Autodesk Inventor part; units mm, degrees
ref_plane "YZ Plane" through (0, 0, 0) normal (1, 0, 0) x (0, 1, 0)
ref_plane "XZ Plane" through (0, 0, 0) normal (0, 1, 0) x (-1, 0, 0)
ref_plane "XY Plane" through (0, 0, 0) normal (0, 0, 1) x (1, 0, 0)
sketch "Sketch1" plane through (0, 0, 0) normal (0, 0, 1) x (1, 0, 0)
  line L0 (0, 0) -> (0, 163.576)
  line L1 (0, 163.576) -> (-73.2155, 163.576)
  line L2 (-73.2155, 163.576) -> (-73.2155, 187.325)
  line L3 (-73.2155, 187.325) -> (-50.8635, 187.325)
  line L4 (-50.8635, 187.325) -> (-50.8635, 260.35)
  line L5 (0, 190.5) -> (0, 163.576)
  line L6 (-50.8635, 260.35) -> (-1.5875, 260.35)
  line L7 (-1.5875, 260.35) -> (-1.5875, 190.5)
  line L8 (-1.5875, 190.5) -> (0, 190.5)
  line L9 (-87.8586, 0) -> (14.6431, 0)
  dimension "d0" = 1.5875
  dimension "d2" = 49.276
  dimension "d3" = 260.35
  dimension "d4" = 190.5
  dimension "d5" = 163.576
  dimension "d6" = 187.325
  dimension "d7" = 71.628
  dimension "d8" = 90
revolve "Revolution1" add sketch "Sketch1" angle 360 about axis through (-10, 0, 0) along (1, 0, 0)
sketch "Sketch2" plane through (0, 0, 0) normal (0, 0, 1) x (1, 0, 0)
  line L0 (-73.2155, -187.325) -> (-73.2155, -163.576)
  line L1 (-73.2155, -163.576) -> (0, -163.576)
  line L2 (0, -163.576) -> (0, -190.5)
  line L3 (0, -190.5) -> (-1.5875, -190.5)
  line L4 (-1.5875, -190.5) -> (-1.5875, -260.35)
  line L5 (-1.5875, -260.35) -> (-50.8635, -260.35)
  line L6 (-50.8635, -260.35) -> (-50.8635, -187.325)
  line L7 (-50.8635, -187.325) -> (-73.2155, -187.325)
  line L8 (-73.2155, 163.576) -> (-73.2155, 187.325)
  line L9 (-73.2155, 187.325) -> (-50.8635, 187.325)
  line L10 (-50.8635, 187.325) -> (-50.8635, 260.35)
  line L11 (-50.8635, 260.35) -> (-1.5875, 260.35)
  line L12 (-1.5875, 260.35) -> (-1.5875, 190.5)
  line L13 (-1.5875, 190.5) -> (0, 190.5)
  line L14 (0, 190.5) -> (0, 163.576)
  line L15 (0, 163.576) -> (-73.2155, 163.576)
  line L16 (0, -190.5) -> (0, 190.5)
  line L17 (0, 165.1) -> (-25.4, 165.1)
  line L18 (-73.2155, 165.1) -> (-73.2155, 166.6875)
  line L19 (-73.2155, 166.6875) -> (-64.6886, 177.8)
  line L20 (-64.6886, 177.8) -> (-60.3885, 177.8)
  line L21 (-50.8635, 177.8) -> (-50.8635, 187.325) construction
  line L22 (0, 165.1) -> (-25.4, 165.1) construction
  line L23 (-25.4, 165.1) -> (-25.4, 160.3375)
  line L24 (-25.4, 160.3375) -> (0, 160.3375)
  line L25 (0, 160.3375) -> (0, 165.1)
  arc A0 (-60.3885, 177.8) -> (-50.8635, 187.325) centre (-60.3885, 187.325) ccw
  line L26 (-60.3885, 177.8) -> (-50.8635, 177.8) construction
  line L27 (-25.4, 165.1) -> (-73.2155, 165.1)
  line L28 (-50.8635, -260.35) -> (-50.8635, 260.35)
  line L29 (-50.8635, 187.325) -> (-50.8635, 260.35)
  line L30 (-50.8635, 260.35) -> (-1.5875, 260.35)
  line L31 (-1.5875, 190.5) -> (0, 190.5)
  line L32 (-87.8586, 0) -> (14.6431, 0)
  point P0 (0, 0)
  dimension "d10" = 1.5875
  dimension "d11" = 37.5
  dimension "d12" = 177.8
  dimension "d13" = 25.4
  dimension "d14" = 160.3375
  dimension "d15" = 165.1
  dimension "d16" = 22.225
revolve "Revolution2" cut sketch "Sketch2" angle 360 about axis through (-10, 0, 0) along (1, 0, 0) contours A0 L20 L19 L8 L9
properties part number "A1-19027-400-06 ALTERNATE TEST FLANGE"
Could you check a few things on this model? Use its own coordinates, in mm. A direction names the side the tool comes from. Give positions to 0.01 mm unless a question says otherwise; leave off trailing zeros. Write each loop counter-clockwise with the first axis right and the second up, starting at its lowest first coordinate (ties: lowest second). Pieces come first, ordered by that corner, then holes. Notation, with made-up numbers: (-7, -13.5) -> (25, -13.5) arc R24 ccw to (25, 3.5) -> close; hole circle Ø9 at (73.5, 13). An arc over 180 degrees is marked (long way). Answer as a JSON object with one key per item and string values.
Q1. Suppose I cut it at C-C on x = -41.5. Write out the boundary of the cut face in (y, z).
Taken from the geometry:
{"outline": "circle Ø520.7 at (0, 0); hole circle Ø327.15 at (0, 0)"}
Q2. Will these pins go through, and if not, where does the flat tip stop? pin 1 Ø4 at (x, z) = (-57.5, -43) entering from +Y; pin 2 Ø10 at (y, z) = (50.5, -184.5) entering from -X; pin 3 Ø5 at (x, z) = (-60.5, -73) entering from -Y.
Taken from the geometry:
{"pin 1": "stops at y = 174.01", "pin 2": "stops at x = -50.92", "pin 3": "stops at y = -163.23"}
Q3. Which directions (+Z, -Z, +X, -X, +Y, -Y) give clear straight access to the entire face, cutting with the end or side of a thin tool? Please do faces 1 (the cylindrical face through (-0.78, -151.17, -115.92)), 2 (the flat face through (-50.864, -177, 62)), 3 (the flat face through (0, 84, 142)).
Taken from the geometry:
{"face 1": "+X", "face 2": "-X", "face 3": "+Z, -Z, +X, +Y, -Y"}
Q4. Please list where these lines run through material, in increasing order: L1, parallel to Z at x = -19, y = 0; L2, parallel to X at y = -21, z = 208.5; L3, parallel to X at y = -130.5, z = 120.5.
Taken from the geometry:
{"L1": "z = -260.35 to -163.58, 163.58 to 260.35", "L2": "x = -50.86 to -1.59", "L3": "x = -64.82 to 0"}
Q5. Suppose I cut it at D-D on y = 210. Write out the boundary of the cut face in (x, z), then the cut area to 3 significant figures.
Taken from the geometry:
{"outline": "(-50.86, -153.89) -> (-1.59, -153.89) -> (-1.59, 153.89) -> (-50.86, 153.89) -> close", "area": "15,200 mm²"}
